```python
from build123d import *

# Parameters (mm, degrees)
CROQUIS2_R              = 5
CROQUIS2_R_2            = 2.5
SALIENTE_EXTRUIR1_DEPTH = 3
CROQUIS3_R              = 4.5
CROQUIS3_R_2            = 3
CORTAR_EXTRUIR1_DEPTH   = 0.5


with BuildPart() as part:
    # Croquis2 → Saliente-Extruir1 (new body)
    with BuildSketch(Plane(origin=(0, 0, 0), x_dir=(1, 0, 0), z_dir=(0, 1, 0))):
        Circle(CROQUIS2_R)
        Circle(CROQUIS2_R_2, mode=Mode.SUBTRACT)
    extrude(amount=SALIENTE_EXTRUIR1_DEPTH)

    # Croquis3 → Cortar-Extruir1 (cut)
    with BuildSketch(Plane(origin=(0, 3, 0), x_dir=(1, 0, 0), z_dir=(0, 1, 0))):
        Circle(CROQUIS3_R)
        Circle(CROQUIS3_R_2, mode=Mode.SUBTRACT)
    cortar_extruir1 = extrude(amount=-CORTAR_EXTRUIR1_DEPTH, mode=Mode.SUBTRACT)

    # Simetría1: Cortar-Extruir1 across plane
    add(cortar_extruir1.mirror(Plane.ZX.offset(1.5)), mode=Mode.SUBTRACT)


solid = part.part
```
Model file for the job. Use its own axes, mm. A direction names the side the tool comes from. Coordinates: 2 decimals unless noted, no trailing zeros. Loops run counter-clockwise (first coordinate to the right, second up) from the corner with the lowest first, then second, coordinate; pieces in that order, holes last. Notation, with made-up numbers: (42.5, 41.5) - (71.5, 41.5) arc R20 cw to (71.5, 54.5) - close; hole circle Ø4 at (88.5, 54). An arc over 180 degrees is marked (long way). Answer as a JSON object with one key per item and string values. Group by question number.
(1) Probe line 1 along X through (y, z) = (0.35, 0); line 2 along X through (y, z) = (1.75, 0). List the from-to ranges inside material, lowest first.
(2) Cut at A-A (x = 0). Give the cut face in (y, z), then the cut area to 3 significant figures.
(3) Tool access for faces 1 (the face through (1, 0.5, 3)), 2 (the face through (-3, 2.8, -0.1)), 3 (the face through (-2, 3, -2)): list every direction of +Z, -Z, +X, -X, +Y, -Y with a clear straight run to the whole face (end or side of a thin tool).
(4) Flat gauge pin, fed straight in: pin 1 (1 mm diameter, centred on y = 1.5, z = -2.5, fed in from -X). Where does the tip first touch, or does it go through?
(5) Two-plate mould, pull along X, no slides. Class faces 4 (the face through (-0.59, 2.75, -4.46)), 5 (the face through (-1.08, 1.48, 4.88)), 6 (the face through (-2, 0, -2)): released by +X, released by -X, zero draft, split by the parting line, or undercut.
(6) Cut at B-B (z = 0). Give the cut face in (x, y).
(7) Cut at D-D (x = 3.75). Give the cut face in (y, z).
(8) Cut at C-C (y = 0.35). Give the cut face in (x, z).
Geometry says:
{
 "1": {"line 1": "x = -5 to -4.5, -3 to -2.5, 2.5 to 3, 4.5 to 5", "line 2": "x = -5 to -2.5, 2.5 to 5"},
 "2": {"outline": "(0, -5) - (3, -5) - (3, -4.5) - (2.5, -4.5) - (2.5, -3) - (3, -3) - (3, -2.5) - (0, -2.5) - (0, -3) - (0.5, -3) - (0.5, -4.5) - (0, -4.5) - close; (0, 2.5) - (3, 2.5) - (3, 3) - (2.5, 3) - (2.5, 4.5) - (3, 4.5) - (3, 5) - (0, 5) - (0, 4.5) - (0.5, 4.5) - (0.5, 3) - (0, 3) - close", "area": "12.0 mm^2"},
 "3": {"face 1": "-Y", "face 2": "+Y", "face 3": "+Z, -Z, +X, -X, +Y"},
 "4": {"pin 1": "stops at x = -4.58"},
 "5": {"face 4": "undercut", "face 5": "split by the parting line", "face 6": "zero draft"},
 "6": {"outline": "(-5, 0) - (-4.5, 0) - (-4.5, 0.5) - (-3, 0.5) - (-3, 0) - (-2.5, 0) - (-2.5, 3) - (-3, 3) - (-3, 2.5) - (-4.5, 2.5) - (-4.5, 3) - (-5, 3) - close; (2.5, 0) - (3, 0) - (3, 0.5) - (4.5, 0.5) - (4.5, 0) - (5, 0) - (5, 3) - (4.5, 3) - (4.5, 2.5) - (3, 2.5) - (3, 3) - (2.5, 3) - close"},
 "7": {"outline": "(0, -3.31) - (3, -3.31) - (3, -2.49) - (2.5, -2.49) - (2.5, 2.49) - (3, 2.49) - (3, 3.31) - (0, 3.31) - (0, 2.49) - (0.5, 2.49) - (0.5, -2.49) - (0, -2.49) - close"},
 "8": {"outline": "circle Ø10 at (0, 0); circle Ø6 at (0, 0); hole circle Ø9 at (0, 0); hole circle Ø5 at (0, 0)"}
}
